from build123d import *

# Parameters (mm, degrees)
F1_DEPTH  = 3
F2_R      = 1.5
F3_DEPTH  = 25
F5_DEPTH  = 4
F6_DEPTH  = 25
F7_R      = 2
F9_DEPTH  = 5
F10_R     = 5
F11_DEPTH = 25


# Not quite as in the source:
# - ends of sketch curves that miss each other by under 0.0002 mm in the source are joined


with BuildPart() as f1:
    # F0 (on Top) → F1 (new body)
    with BuildSketch(Plane.XY):
        with BuildLine():
            ThreePointArc((49.2280806434, 33.0130470502), (48.1713658013, 32.5621821126), (47.1108383201, 32.1203598507))
            Line((47.1108383201, 32.1203598507), (-4.1065374511, -22.3721440377))
            Line((-4.1065374511, -22.3721440377), (54.4172076095, -84.5927516487))
            Line((54.4172076095, -84.5927516487), (54.4172076095, 33.0130470502))
            Line((54.4172076095, 33.0130470502), (49.2280806434, 33.0130470502))
        make_face()
        Polygon((-4.1065374511, -22.3721440377), (-62.5827923905, -84.587700803), (-62.5827923905, -85.003347494), (54.4172076095, -85.003347494), (54.4172076095, -84.5927516487), align=None)
        with BuildLine():
            Line((-62.5827923905, 33.0130470502), (-62.5827923905, -84.587700803))
            Line((-62.5827923905, -84.587700803), (-4.1065374511, -22.3721440377))
            Line((-4.1065374511, -22.3721440377), (-55.4151337668, 32.1775440438))
            ThreePointArc((-55.4151337668, 32.1775440438), (-56.406067296, 32.5913463114), (-57.3936654243, 33.0130470502))
            Line((-57.3936654243, 33.0130470502), (-62.5827923905, 33.0130470502))
        make_face()
        with BuildLine():
            Line((-4.1065374511, -22.3721440377), (47.1108383201, 32.1203598507))
            ThreePointArc((47.1108383201, 32.1203598507), (-4.1578101896, 21.9966734267), (-55.4151337668, 32.1775440438))
            Line((-55.4151337668, 32.1775440438), (-4.1065374511, -22.3721440377))
        make_face()
        with BuildLine():
            ThreePointArc((60.9172316623, 46.8096119171), (-4.082778411, 28.996652506), (-69.0827923905, 46.8095976636))
            Line((-69.0827923905, 46.8095976636), (-69.0827923905, -91.503347494))
            Line((-69.0827923905, -91.503347494), (-62.5827923905, -84.587700803))
            Line((-62.5827923905, -84.587700803), (-62.5827923905, 33.0130470502))
            Line((-62.5827923905, 33.0130470502), (-57.3936654243, 33.0130470502))
            ThreePointArc((-57.3936654243, 33.0130470502), (-56.406067296, 32.5913463114), (-55.4151337668, 32.1775440438))
            ThreePointArc((-55.4151337668, 32.1775440438), (-4.1578101896, 21.9966734267), (47.1108383201, 32.1203598507))
            Line((47.1108383201, 32.1203598507), (60.9172316623, 46.8096119171))
        make_face()
        with BuildLine():
            Line((60.9172076095, -91.503347494), (60.9172076095, 46.809652506))
            Line((60.9172076095, 46.809652506), (47.1108383201, 32.1203598507))
            ThreePointArc((47.1108383201, 32.1203598507), (48.1713658013, 32.5621821126), (49.2280806434, 33.0130470502))
            Line((49.2280806434, 33.0130470502), (54.4172076095, 33.0130470502))
            Line((54.4172076095, 33.0130470502), (54.4172076095, -84.5927516487))
            Line((54.4172076095, -84.5927516487), (60.9172076095, -91.503347494))
        make_face()
        Polygon((-62.5827923905, -84.587700803), (-69.0827923905, -91.503347494), (60.9172076095, -91.503347494), (54.4172076095, -84.5927516487), (54.4172076095, -85.003347494), (-62.5827923905, -85.003347494), align=None)
    extrude(amount=F1_DEPTH)

    # F2 (on face) → F3 (cut)
    with BuildSketch(Plane.XY.offset(3)):
        with Locations((58.4172076095, -76.503347494)):
            Circle(F2_R)
        with Locations((58.4172076095, -26.503347494)):
            Circle(F2_R)
        with Locations((58.4172076095, 23.496652506)):
            Circle(F2_R)
        with Locations((-4.0827923905, 26.496652506)):
            Circle(F2_R)
        with Locations((-66.5827923905, -76.503347494)):
            Circle(F2_R)
        with Locations((-4.0827923905, -89.003347494)):
            Circle(F2_R)
        with Locations((-66.5827923905, -26.503347494)):
            Circle(F2_R)
        with Locations((-66.5827923905, 23.496652506)):
            Circle(F2_R)
    extrude(amount=-F3_DEPTH, mode=Mode.SUBTRACT)

    # F4 (on face) → F5 (join)
    with BuildSketch(Plane.XY.offset(3)):
        with BuildLine():
            Line((-13.011363819, -40.0015251468), (-13.011363819, -22.5051698412))
            ThreePointArc((-13.011363819, -22.5051698412), (-16.5827923905, -31.253347494), (-13.011363819, -40.0015251468))
        make_face()
        with BuildLine():
            ThreePointArc((4.8457790381, -40.0015251468), (7.4899588567, -35.9779034066), (8.4172076095, -31.253347494))
            ThreePointArc((8.4172076095, -31.253347494), (7.4899588567, -26.5287915814), (4.8457790381, -22.5051698412))
            Line((4.8457790381, -22.5051698412), (4.8457790381, -40.0015251468))
        make_face()
        with BuildLine():
            Line((1.2743504667, -42.5471962803), (1.2743504667, -19.9594987077))
            ThreePointArc((1.2743504667, -19.9594987077), (-0.4709241544, -19.2865430816), (-2.2970781048, -18.8815560114))
            Line((-2.2970781048, -18.8815560114), (-2.2970781048, -43.6251389767))
            ThreePointArc((-2.2970781048, -43.6251389767), (-0.4709241544, -43.2201519064), (1.2743504667, -42.5471962803))
        make_face()
        with BuildLine():
            Line((-5.8685066762, -43.6251389767), (-5.8685066762, -18.8815560114))
            ThreePointArc((-5.8685066762, -18.8815560114), (-7.6946606266, -19.2865430816), (-9.4399352476, -19.9594987077))
            Line((-9.4399352476, -19.9594987077), (-9.4399352476, -42.5471962803))
            ThreePointArc((-9.4399352476, -42.5471962803), (-7.6946606266, -43.2201519064), (-5.8685066762, -43.6251389767))
        make_face()
    extrude(amount=F5_DEPTH)

    # F4 (on face) → F6 (cut)
    with BuildSketch(Plane.XY.offset(3)):
        with BuildLine():
            Line((-9.4399352476, -42.5471962803), (-9.4399352476, -19.9594987077))
            ThreePointArc((-9.4399352476, -19.9594987077), (-11.3381709845, -21.0744732215), (-13.011363819, -22.5051698412))
            Line((-13.011363819, -22.5051698412), (-13.011363819, -40.0015251468))
            ThreePointArc((-13.011363819, -40.0015251468), (-11.3381709845, -41.4322217666), (-9.4399352476, -42.5471962803))
        make_face()
        with BuildLine():
            Line((-2.2970781048, -43.6251389767), (-2.2970781048, -18.8815560114))
            ThreePointArc((-2.2970781048, -18.8815560114), (-4.0827923905, -18.753347494), (-5.8685066762, -18.8815560114))
            Line((-5.8685066762, -18.8815560114), (-5.8685066762, -43.6251389767))
            ThreePointArc((-5.8685066762, -43.6251389767), (-4.0827923905, -43.753347494), (-2.2970781048, -43.6251389767))
        make_face()
        with BuildLine():
            Line((4.8457790381, -40.0015251468), (4.8457790381, -22.5051698412))
            ThreePointArc((4.8457790381, -22.5051698412), (3.1725862036, -21.0744732215), (1.2743504667, -19.9594987077))
            Line((1.2743504667, -19.9594987077), (1.2743504667, -42.5471962803))
            ThreePointArc((1.2743504667, -42.5471962803), (3.1725862036, -41.4322217666), (4.8457790381, -40.0015251468))
        make_face()
    extrude(amount=-F6_DEPTH, mode=Mode.SUBTRACT)

    # F7
    f7_edges = [f1.edges().sort_by_distance(p)[0] for p in [
        (-7.694661, -19.286543, 7),
        (-16.582792, -31.253347, 7),
        (-0.470924, -19.286543, 7),
        (8.417208, -31.253347, 7),
        (-0.470924, -43.220152, 7),
        (-7.694661, -43.220152, 7),
    ]]
    fillet(f7_edges, radius=F7_R)

    # F8 (on face) → F9 (cut)
    with BuildSketch(Plane(origin=(0, 0, 0), x_dir=(1, 0, 0), z_dir=(0, 0, -1))):
        with BuildLine():
            ThreePointArc((4.8457790381, 24.5226173164), (6.3865506098, 27.5722856522), (6.9172076095, 30.9476163238))
            ThreePointArc((6.9172076095, 30.9476163238), (6.3865506098, 34.3229469955), (4.8457790381, 37.3726153312))
            Line((4.8457790381, 37.3726153312), (4.8457790381, 24.5226173164))
        make_face()
        with BuildLine():
            Line((1.2743504667, 21.3402743185), (1.2743504667, 40.5549583292))
            ThreePointArc((1.2743504667, 40.5549583292), (-0.4573688452, 41.3330052967), (-2.2970781048, 41.8017042399))
            Line((-2.2970781048, 41.8017042399), (-2.2970781048, 20.0935284078))
            ThreePointArc((-2.2970781048, 20.0935284078), (-0.4573688452, 20.562227351), (1.2743504667, 21.3402743185))
        make_face()
        with BuildLine():
            Line((-2.2970781048, 20.0935284078), (-2.2970781048, 41.8017042399))
            ThreePointArc((-2.2970781048, 41.8017042399), (-4.0827923905, 41.9476163238), (-5.8685066762, 41.8017042399))
            Line((-5.8685066762, 41.8017042399), (-5.8685066762, 20.0935284078))
            ThreePointArc((-5.8685066762, 20.0935284078), (-4.0827923905, 19.9476163238), (-2.2970781048, 20.0935284078))
        make_face()
        with BuildLine():
            Line((-5.8685066762, 20.0935284078), (-5.8685066762, 41.8017042399))
            ThreePointArc((-5.8685066762, 41.8017042399), (-7.7082159357, 41.3330052967), (-9.4399352476, 40.5549583292))
            Line((-9.4399352476, 40.5549583292), (-9.4399352476, 21.3402743185))
            ThreePointArc((-9.4399352476, 21.3402743185), (-7.7082159357, 20.562227351), (-5.8685066762, 20.0935284078))
        make_face()
        with BuildLine():
            Line((-9.4399352476, 21.3402743185), (-9.4399352476, 40.5549583292))
            ThreePointArc((-9.4399352476, 40.5549583292), (-11.4007316429, 39.1602751562), (-13.011363819, 37.3726153312))
            Line((-13.011363819, 37.3726153312), (-13.011363819, 24.5226173164))
            ThreePointArc((-13.011363819, 24.5226173164), (-11.4007316429, 22.7349574914), (-9.4399352476, 21.3402743185))
        make_face()
        with BuildLine():
            Line((-13.011363819, 24.5226173164), (-13.011363819, 37.3726153312))
            ThreePointArc((-13.011363819, 37.3726153312), (-15.0827923905, 30.9476163238), (-13.011363819, 24.5226173164))
        make_face()
    extrude(amount=-F9_DEPTH, mode=Mode.SUBTRACT)

    # F10 (on face) → F11 (cut)
    with BuildSketch(Plane.XY.offset(3)):
        with Locations((-4.0827923905, -61.503347494)):
            Circle(F10_R)
    extrude(amount=-F11_DEPTH, mode=Mode.SUBTRACT)


solid = f1.part
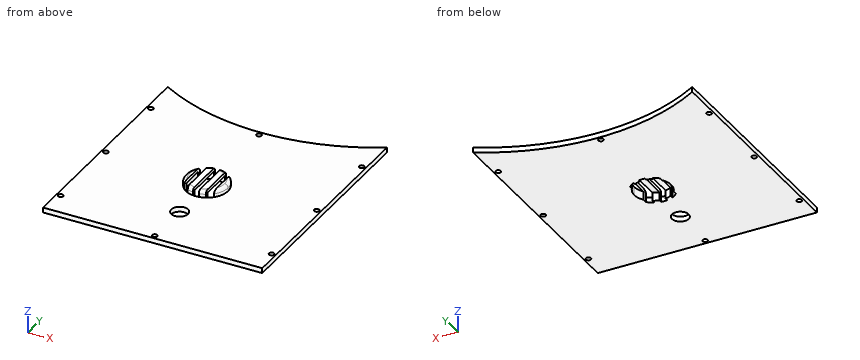
Can you work these out from the model? Positions are in its coordinate system, mm. Coordinates: 2 decimals unless noted, no trailing zeros. Write each loop counter-clockwise with the first axis right and the second up, starting at its lowest first coordinate (ties: lowest second). Pieces come first, ordered by that corner, then holes.
Q1. For P1, Ø1.7, axis at x = -13.5, y = -32.5, coming from the -Z side; P2, Ø5, axis at x = -3, y = -62.5, coming from the +Z side; P3, Ø4, axis at x = -4.08, y = -89, coming from the +Z side, each with a flat end and sliding along its axis, tell me the tip position at first contact or that it passes through.
Results found:
P1: stops at z = 5
P2: passes through
P3: stops at z = 3
Q2. Imagine slicing it at B-B, the plane x = -52. List the corners of the cut face in (y, z) for me.
Results found:
outline: (-91.5, 0) - (38.34, 0) - (38.34, 3) - (-91.5, 3) - close
Q3. Please list where these lines run through material, in increasing order: L1, parallel to X at y = -29, z = 5.25; L2, parallel to X at y = -20.5, z = 6.25; L3, parallel to X at y = -32, z = 5.5.
Results found:
L1: x = -16.36 to -13.01, -9.44 to -5.87, -2.3 to 1.27, 4.85 to 8.2
L2: x = -9.44 to -5.87, -2.3 to 1.27
L3: x = -16.5 to -13.01, -9.44 to -5.87, -2.3 to 1.27, 4.85 to 8.33
Q4. Imagine slicing it at A-A, the plane y = -16.5. List the corners of the cut face in (x, z) for me.
Results found:
outline: (-69.08, 0) - (60.92, 0) - (60.92, 3) - (-69.08, 3) - close
